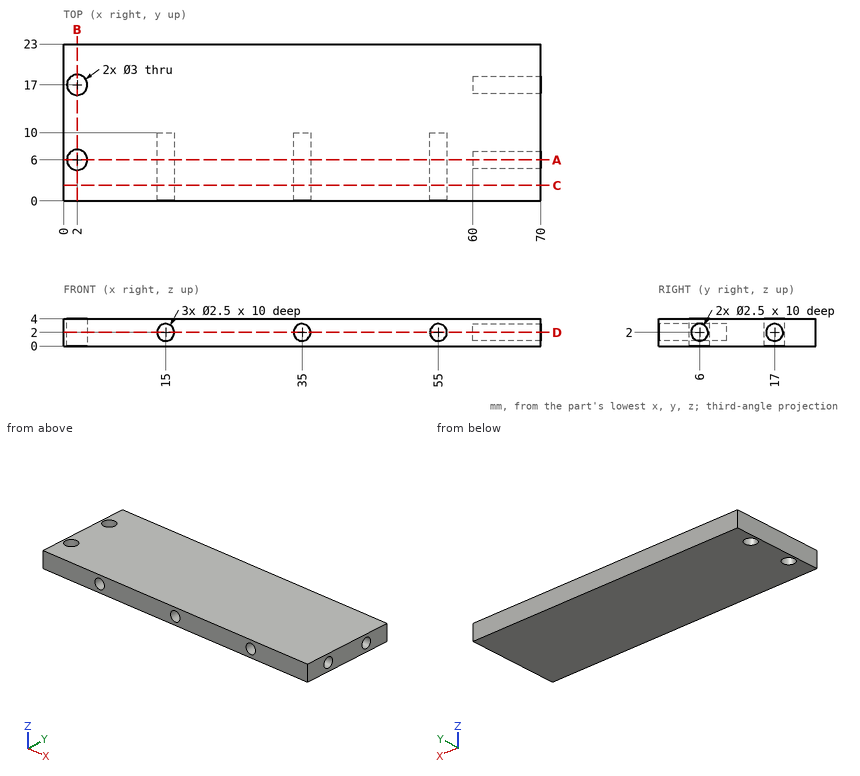
Check sheet for the drawn part. Datum: minimum x, y, z corner. Units: mm. Give positions to 0.01 mm unless a question says otherwise; leave off trailing zeros. Order: outer loops, then holes, each group sorted by start corner. A loop starts at its lowest first (then second) coordinate and runs counter-clockwise, first axis right, second up.
1. Sectioned sample at A-A (y = 6). Record the boundary of the cut face in (x, z), then the cut area to 3 significant figures.
Completed:
outline: (0, 0) - (0.5, 0) - (0.5, 4) - (0, 4) - close; (3.5, 0) - (70, 0) - (70, 0.75) - (60, 0.75) - (60, 3.25) - (70, 3.25) - (70, 4) - (3.5, 4) - close; hole circle Ø2.5 at (15, 2); hole circle Ø2.5 at (35, 2); hole circle Ø2.5 at (55, 2)
area: 228 mm2
2. Depth check by flat-ended pin: pin 1 (0.8 mm diameter, centred on y = 6, z = 2, fed in from +X); pin 2 (2.5 mm diameter, centred on x = 2, y = 6, fed in from +Z); pin 3 (0.8 mm diameter, centred on x = 34.5, z = 2, fed in from -Y). Enter the tip coordinate at first touch or a pass-through.
Completed:
pin 1: stops at x = 60
pin 2: passes through
pin 3: stops at y = 10
3. Sectioned sample at C-C (y = 2.25). Record the boundary of the cut face in (x, z).
Completed:
outline: (0, 0) - (70, 0) - (70, 4) - (0, 4) - close; hole circle Ø2.5 at (15, 2); hole circle Ø2.5 at (35, 2); hole circle Ø2.5 at (55, 2)
4. Sectioned sample at B-B (x = 2). Record the boundary of the cut face in (y, z), then the cut area to 3 significant figures.
Completed:
outline: (0, 0) - (4.5, 0) - (4.5, 4) - (0, 4) - close; (7.5, 0) - (15.5, 0) - (15.5, 4) - (7.5, 4) - close; (18.5, 0) - (23, 0) - (23, 4) - (18.5, 4) - close
area: 68.0 mm2
5. Sectioned sample at D-D (z = 2). Record the boundary of the cut face in (x, y).
Completed:
outline: (0, 0) - (13.75, 0) - (13.75, 10) - (16.25, 10) - (16.25, 0) - (33.75, 0) - (33.75, 10) - (36.25, 10) - (36.25, 0) - (53.75, 0) - (53.75, 10) - (56.25, 10) - (56.25, 0) - (70, 0) - (70, 4.75) - (60, 4.75) - (60, 7.25) - (70, 7.25) - (70, 15.75) - (60, 15.75) - (60, 18.25) - (70, 18.25) - (70, 23) - (0, 23) - close; hole circle Ø3 at (2, 6); hole circle Ø3 at (2, 17)
6. Scan lines: line 1 (X direction, y = 2.5, z = 2); line 2 (Y direction, x = 67, z = 2); line 3 (X direction, y = 6.75, z = 2). Record each from-to range of solid material in increasing order.
Completed:
line 1: x = 0 to 13.75, 16.25 to 33.75, 36.25 to 53.75, 56.25 to 70
line 2: y = 0 to 4.75, 7.25 to 15.75, 18.25 to 23
line 3: x = 0 to 0.7, 3.3 to 13.75, 16.25 to 33.75, 36.25 to 53.75, 56.25 to 60
